The model under review builds one solid part; all positions refer to its coordinate system, in mm. A direction names the side the tool comes from. Coordinates: 2 decimals unless noted, no trailing zeros. Write each loop counter-clockwise with the first axis right and the second up, starting at its lowest first coordinate (ties: lowest second). Pieces come first, ordered by that corner, then holes.
1) Mouldability with a two-part tool opening along X and no side actions: class faces 3 (the cylindrical face through (11.923, 3.755, 9.86)), 4 (the flat face through (7.381, 0, 13)), 5 (the flat face through (-0.2, -5.4, 0)) as released by +X, released by -X, zero draft, split by the parting line, or undercut.
2) For line 1 (X direction, y = -0.25, z = 16.25); line 2 (Y direction, x = 5.75, z = 10.5); line 3 (Y direction, x = -6.75, z = 23.5), list the stretches that pass through material, from the lowest coordinate up.
3) Add section B-B, the plane z = 3.5. State the section outline as (x, y) points, then the cut area to 3 significant figures.
4) Machinability: for faces 1 (the flat face through (-8.539, 0, 13)), 2 (the flat face through (0, 6, 25)), which of the approach directions +Z, -Z, +X, -X, +Y, -Y give a long, thin tool a straight path to every point of the face, cutting with its end or side? Answer none if there is none.
5) For P1, Ø1.5, axis at x = 8.5, y = -2.5, coming from the +Z side; P2, Ø5, axis at y = -4, z = 19, coming from the +X side; P3, Ø4, axis at x = -6.5, z = 6.5, coming from the -Y side, all flat-tipped, find the tip position at first contact; note any pin that passes through.
6) Add section A-A, the plane y = 0. State the section outline as (x, z) points, then the cut area to 3 significant figures.
7) Add section C-C, the plane x = 0. State the section outline as (y, z) points.
from build123d import *

# Parameters (mm, degrees)
F0_R     = 12.5
F1_DEPTH = 25
F2_W     = 15.9198134206
F2_H     = 10.5606685393
F3_DEPTH = 25


# Not quite as in the source:
# - a fillet or chamfer that OpenCascade refuses, or shapes differently, is made with other operations: its cross-section is extruded or revolved along the edge and cut away or added


with BuildPart() as f1:
    # F0 (on Top) → F1 (new body)
    with BuildSketch(Plane.XY):
        Circle(F0_R)
    extrude(amount=F1_DEPTH)

    # F2 (on face) → F3 (cut)
    with BuildSketch(Plane.XY.offset(25)):
        with Locations((-0.578898238, 0.2196121495)):
            Rectangle(F2_W, F2_H)
    extrude(amount=-F3_DEPTH, mode=Mode.SUBTRACT)

    # F4: fillet of radius 5 on 1 edges, made by hand

    # F4_s1 → F4_t2 (revolve, cut)
    with BuildSketch(Plane.XZ):
        with BuildLine():
            ThreePointArc((12.5, 20), (11.0355339059, 23.5355339059), (7.5, 25))
            Line((7.5, 25), (12.5, 25))
            Line((12.5, 25), (12.5, 20))
        make_face()
    revolve(axis=Axis((0, 0, 25), (0, 0, 1)), mode=Mode.SUBTRACT)


solid = f1.part
Geometry results:
1. face 3: split by the parting line
1. face 4: undercut
1. face 5: zero draft
2. line 1: x = -12.5 to -8.54, 7.38 to 12.5
2. line 2: y = -11.1 to -5.06, 5.5 to 11.1
2. line 3: y = -8.77 to -5.06, 5.5 to 8.77
3. outline: circle Ø25 at (0, 0); hole (-8.54, -5.06) - (7.38, -5.06) - (7.38, 5.5) - (-8.54, 5.5) - close
3. area: 323 mm2
4. face 1: +Z, -Z
4. face 2: +Z, +X, -X, +Y, -Y
5. P1: stops at z = 24.96
5. P2: stops at x = 12.41
5. P3: stops at y = -11.66
6. outline: (-12.5, 0) - (-8.54, 0) - (-8.54, 24.89) arc R5 ccw to (-12.5, 20) - close; (7.38, 0) - (12.5, 0) - (12.5, 20) arc R5 ccw to (7.5, 25) - (7.38, 25) - close
6. area: 216 mm2
7. outline: (-12.5, 0) - (-5.06, 0) - (-5.06, 25) - (-7.5, 25) arc R5 ccw to (-12.5, 20) - close; (5.5, 0) - (12.5, 0) - (12.5, 20) arc R5 ccw to (7.5, 25) - (5.5, 25) - close
